Study the drawing (mm; zero at the part's minimum x, y, z) and answer. Coordinates: 2 decimals unless noted, no trailing zeros. Loops run counter-clockwise (first coordinate to the right, second up) from the corner with the lowest first, then second, coordinate; pieces in that order, holes last. Notation, with made-up numbers: (46.5, 4.5) -> (66.5, 4.5) arc R25 cw to (66.5, 41.5) -> close; hole circle Ø2 at (56.25, 0). An arc over 180 degrees is marked (long way). One line per question, with ' | ' between items.
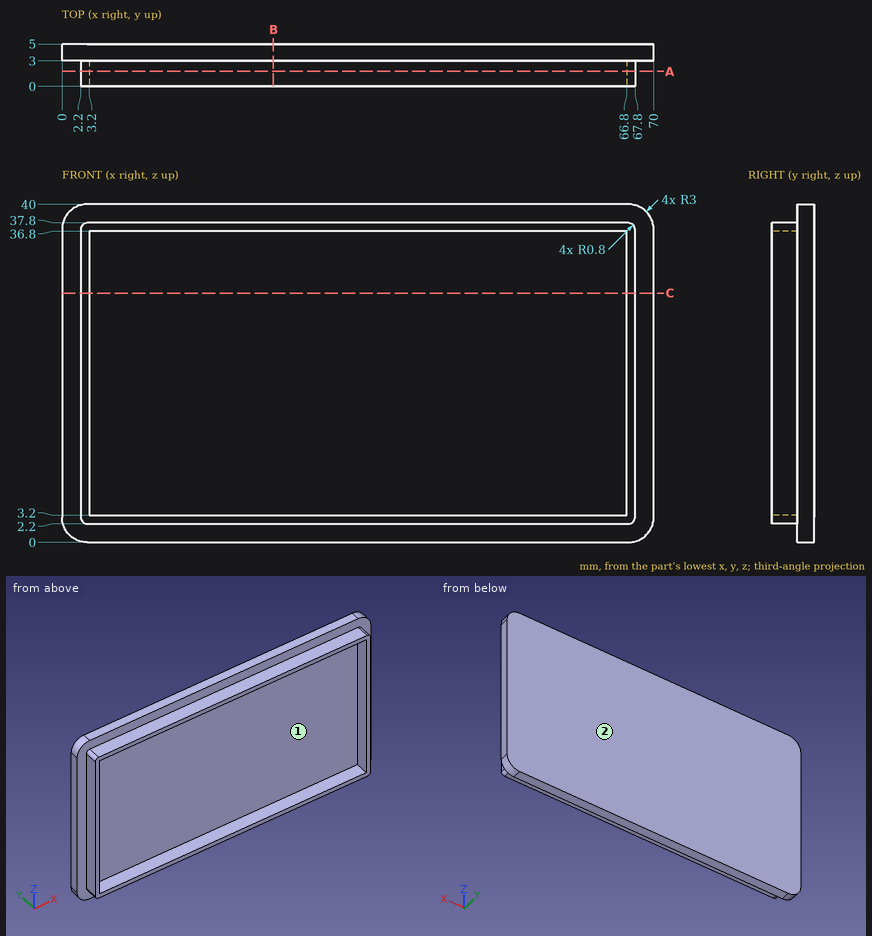
1) The mould has two halves that part along X. Classify the marked faces 1 and 2: released by +X, released by -X, zero draft, split by the parting line, or undercut.
Check values:
face 1: undercut | face 2: zero draft
2) Find the intervals of material crossed by line 1 along X through (y, z) = (1.5, 11); line 2 along Z through (x, y) = (35.5, 2.7); line 3 along Y through (x, z) = (58.5, 33), in increasing order.
Check values:
line 1: x = 2.2 to 3.2, 66.8 to 67.8 | line 2: z = 2.2 to 3.2, 36.8 to 37.8 | line 3: y = 3 to 5
3) Flat-ended cylindrical pins translate along their axes: pin 1 (4 mm diameter, centred on x = 49.5, z = 18, fed in from -Y); pin 2 (0.9 mm diameter, centred on y = 1.5, z = 18, fed in from +X); pin 3 (2.5 mm diameter, centred on x = 45, y = 1.5, fed in from +Z). Find the tip coordinate at first contact, or state that the pin passes through.
Check values:
pin 1: stops at y = 3 | pin 2: stops at x = 67.8 | pin 3: stops at z = 37.8
4) Find section B-B (x = 25). Write down the section's boundary in (y, z), plus the area to 3 significant figures.
Check values:
outline: (0, 2.2) -> (3, 2.2) -> (3, 0) -> (5, 0) -> (5, 40) -> (3, 40) -> (3, 37.8) -> (0, 37.8) -> (0, 36.8) -> (3, 36.8) -> (3, 3.2) -> (0, 3.2) -> close | area: 86.0 mm^2
5) Find section A-A (y = 1.75). Write down the section's boundary in (x, z), plus the area to 3 significant figures.
Check values:
outline: (2.2, 3) arc R0.8 ccw to (3, 2.2) -> (67, 2.2) arc R0.8 ccw to (67.8, 3) -> (67.8, 37) arc R0.8 ccw to (67, 37.8) -> (3, 37.8) arc R0.8 ccw to (2.2, 37) -> close; hole (3.2, 3.2) -> (66.8, 3.2) -> (66.8, 36.8) -> (3.2, 36.8) -> close | area: 198 mm^2
6) Find section C-C (z = 29.5). Write down the section's boundary in (x, y).
Check values:
outline: (0, 3) -> (2.2, 3) -> (2.2, 0) -> (3.2, 0) -> (3.2, 3) -> (66.8, 3) -> (66.8, 0) -> (67.8, 0) -> (67.8, 3) -> (70, 3) -> (70, 5) -> (0, 5) -> close
